Input: dimensioned drawing with shaded views. Units: mm. Origin: part minimum x, y, z. Coordinates: 2 decimals unless noted, no trailing zeros. Loops run counter-clockwise (first coordinate to the right, second up) from the corner with the lowest first, then second, coordinate; pieces in that order, holes last. Notation, with made-up numbers: (67, -13) -> (99, -13) arc R32 ccw to (99, 20) -> close; hole circle Ø10 at (31.25, 66). An arc over 180 degrees is marked (long way). Answer as CSV lines item,"result".
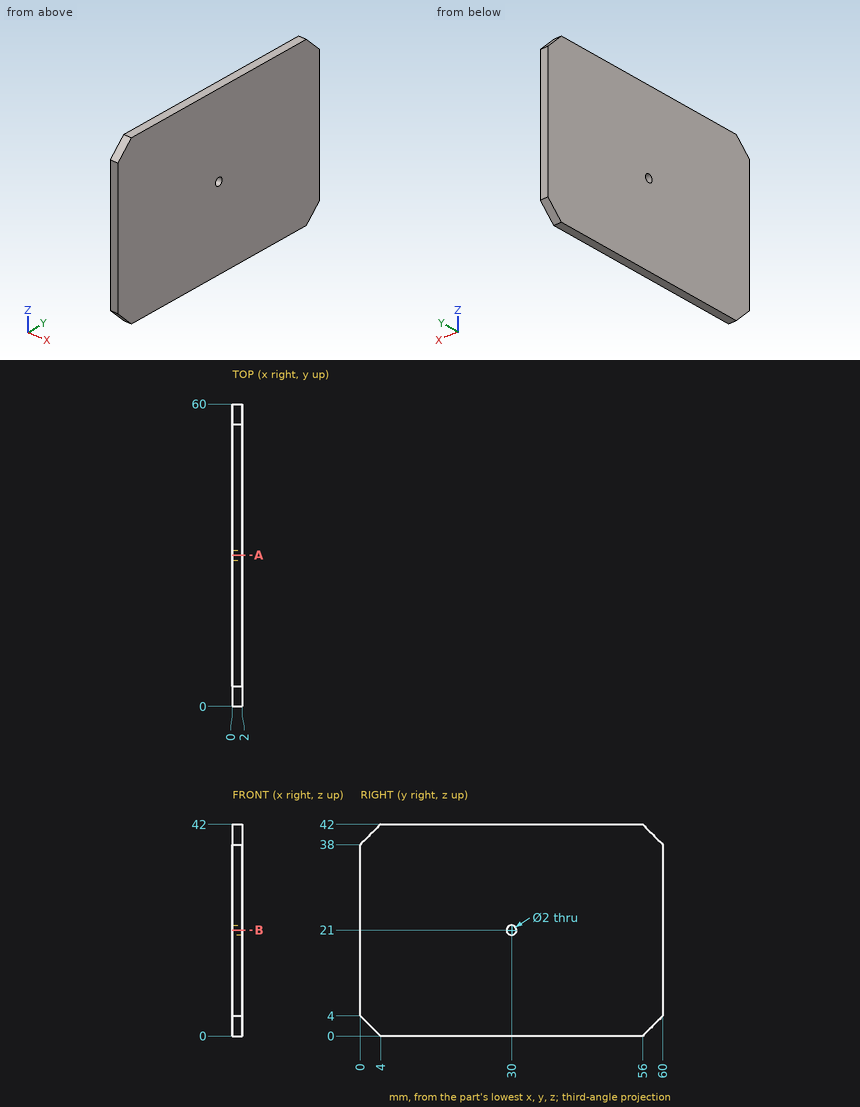
(1) Material intervals for L1, parallel to Y at x = 0.75, z = 21; L2, parallel to Z at x = 1, y = 30.5, sorted ascending. Write a range as [from, to].
Computed values:
L1,"[0, 29], [31, 60]"
L2,"[0, 20.13], [21.87, 42]"
(2) Pin query (flat end, axial travel): pin 1 Ø1.2 at (y, z) = (30, 21) entering from +X. Return the tip coordinate at first contact, or that it passes through.
Computed values:
pin 1,"through"
(3) Cut plane A-A (y = 30). Return the cut outline in (x, z), then the cut area to 3 significant figures.
Computed values:
outline,"(0, 0) -> (2, 0) -> (2, 20) -> (0, 20) -> close; (0, 22) -> (2, 22) -> (2, 42) -> (0, 42) -> close"
area,"80.0 mm^2"
(4) Cut plane B-B (z = 21). Return the cut outline in (x, y), then the cut area to 3 significant figures.
Computed values:
outline,"(0, 0) -> (2, 0) -> (2, 29) -> (0, 29) -> close; (0, 31) -> (2, 31) -> (2, 60) -> (0, 60) -> close"
area,"116 mm^2"
